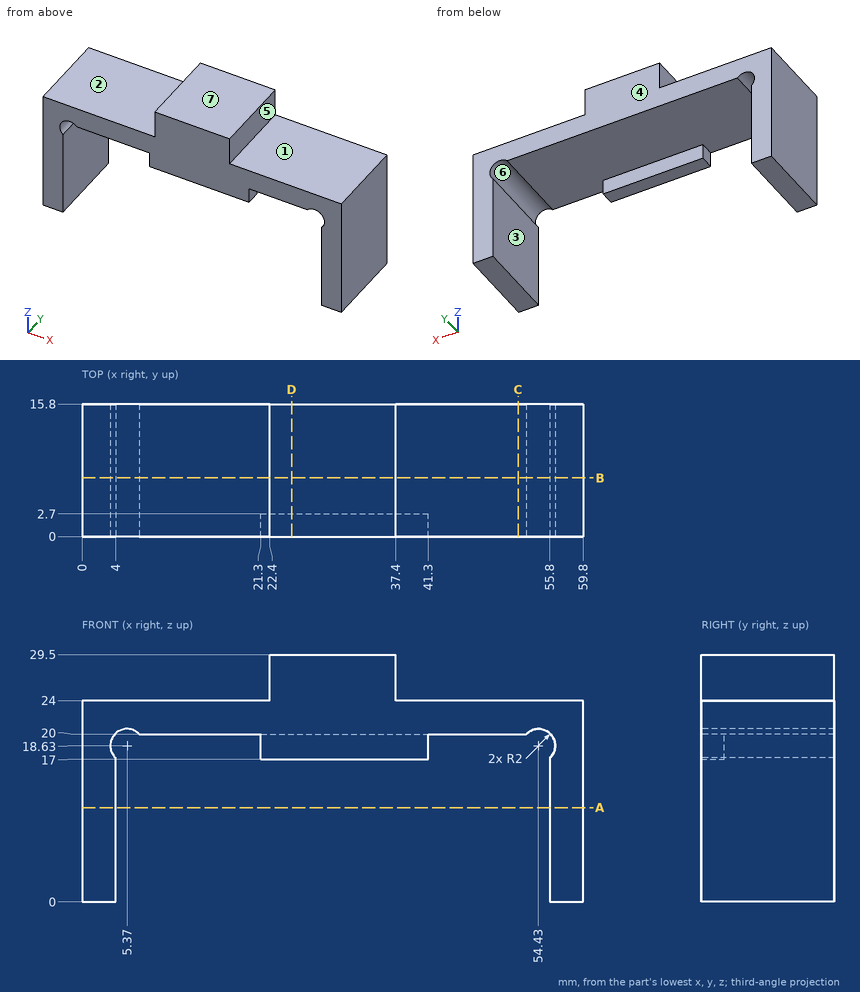
Study the drawing (mm; zero at the part's minimum x, y, z) and answer. A direction names the side the tool comes from. Coordinates: 2 decimals unless noted, no trailing zeros. Loops run counter-clockwise (first coordinate to the right, second up) from the corner with the lowest first, then second, coordinate; pieces in that order, holes last. Notation, with made-up numbers: (86, 34) -> (125, 34) arc R11 cw to (125, 49) -> close; hole circle Ø1 at (-39, 11). An arc over 180 degrees is marked (long way). Write each question's results on one line, items separated by ' | '. Start each with the question number.
1) Flat-ended cylindrical pins translate along their axes: P1, Ø0.9, axis at x = 35, z = 18, coming from the +Y side; P2, Ø1, axis at y = 14, z = 25, coming from the +X side; P3, Ø4.5, axis at x = 47.5, y = 11.5, coming from the +Z side; P4, Ø5, axis at x = 33, z = 14, coming from the -Y side. Find the tip coordinate at first contact, or state that the pin passes through.
2) Find section C-C on x = 52. Determine the outline of the cut face in (y, z).
3) Find section A-A on z = 11.25. Determine the outline of the cut face in (x, y).
4) The mould has two halves that part along Z. Classify the marked faces 5, 6 and 7: pulls with the +Z half, pulls with the -Z half, needs draft (parallel to the pull), parting line crosses it, or undercut.
5) Consider line 1 along X through (y, z) = (6.75, 2.5); line 2 along Z through (x, y) = (22.5, 6.25); line 3 along X through (y, z) = (10, 27.25). Determine where each line is inside the solid, lowest interval first.
6) For the marked faces 1, 2, 3 and 4, determine the directions among +Z, -Z, +X, -X, +Y, -Y from which every point of the face is accessible in a straight line to the end or side of a thin tool.
7) Find section D-D on x = 25. Determine the outline of the cut face in (y, z).
8) Find section B-B on y = 7. Determine the outline of the cut face in (x, z), then the cut area to 3 significant figures.
Response values:
1) P1: stops at y = 2.7 | P2: stops at x = 37.4 | P3: stops at z = 24 | P4: passes through
2) outline: (0, 20) -> (15.8, 20) -> (15.8, 24) -> (0, 24) -> close
3) outline: (0, 0) -> (4, 0) -> (4, 15.8) -> (0, 15.8) -> close; (55.8, 0) -> (59.8, 0) -> (59.8, 15.8) -> (55.8, 15.8) -> close
4) face 5: needs draft | face 6: undercut | face 7: pulls with the +Z half
5) line 1: x = 0 to 4, 55.8 to 59.8 | line 2: z = 20 to 29.5 | line 3: x = 22.4 to 37.4
6) face 1: +Z, +X, +Y, -Y | face 2: +Z, -X, +Y, -Y | face 3: -Z, +Y, -Y | face 4: +Z, -Z, +X, -X, +Y
7) outline: (0, 17) -> (2.7, 17) -> (2.7, 20) -> (15.8, 20) -> (15.8, 29.5) -> (0, 29.5) -> close
8) outline: (0, 0) -> (4, 0) -> (4, 17.17) arc R2 cw (long way) to (6.83, 20) -> (52.97, 20) arc R2 cw (long way) to (55.8, 17.17) -> (55.8, 0) -> (59.8, 0) -> (59.8, 24) -> (37.4, 24) -> (37.4, 29.5) -> (22.4, 29.5) -> (22.4, 24) -> (0, 24) -> close | area: 477 mm^2
